Input: part model. Units: mm. Frame: model coordinates. Face numbers are marked on the shaded views. Coordinates: 2 decimals unless noted, no trailing zeros. Loops run counter-clockwise (first coordinate to the right, second up) from the corner with the lowest first, then second, coordinate; pieces in that order, holes last.
(1) Section C-C, the plane y = 4. Return loops of the section in (x, z).
(2) Line query: L1, parallel to X at y = 6.5, z = 0; L2, parallel to Z at x = 41, y = 5.25; L3, parallel to Z at x = 16.5, y = 4.75. Output: solid intervals per line, ascending.
(3) Contact query for flat-ended pins moving along their axis: P1, Ø1.5, axis at x = 13.5, y = 2.5, coming from the +Z side; P2, Ø2, axis at x = 41, z = 0, coming from the +Y side; P3, Ø5, axis at y = 7, z = 2, coming from the -X side; P4, Ø3, axis at x = -14.5, y = 3, coming from the -Z side. Output: stop coordinate, or through.
(4) Section B-B, the plane x = -14.5. Return loops of the section in (y, z), then the cut area to 3 significant figures.
(5) Mould query, pull axis X, two halves, no side actions, for the marked faces 1, 2 and 3. Classes: released by +X, released by -X, zero draft, split by the parting line, or undercut.
(6) Section A-A, the plane z = -16. Return loops of the section in (x, y).
(7) Section D-D, the plane x = -41. Return loops of the section in (y, z).
```python
from build123d import *

# Parameters (mm, degrees)
SCHIZZO1_R                             = 47
SCHIZZO1_R_2                           = 35
ESTRUSIONE_ESTRUSIONE1_DEPTH           = 10
FORO_SVASATO_PER_VITE_M3_1_D           = 3.4
FORO_SVASATO_PER_VITE_M3_1_DEPTH       = 188
FORO_SVASATO_PER_VITE_M3_1_CSINK_D     = 6.3
FORO_SVASATO_PER_VITE_M3_1_CSINK_ANGLE = 90
FORO_SVASATO_PER_VITE_M3_1_TIP         = 1.021463052


with BuildPart() as part:
    # Schizzo1 → Estrusione-Estrusione1 (new body)
    with BuildSketch(Plane(origin=(0, 0, 0), x_dir=(1, 0, 0), z_dir=(0, 1, 0))):
        with Locations(Location((0, 0, 0), (0, 0, 270))):
            Circle(SCHIZZO1_R)
        with Locations(Location((0, 0, 0), (0, 0, 270))):
            Circle(SCHIZZO1_R_2, mode=Mode.SUBTRACT)
    extrude(amount=ESTRUSIONE_ESTRUSIONE1_DEPTH)

    # Foro svasato per Vite M3-1
    with Locations(Plane(origin=(-41, 10, 0), x_dir=(0, 0, 1), z_dir=(0, 1, 0))):
        with Locations((0, 0), (0, 82), (41, 41), (-41, 41)):
            CounterSinkHole(FORO_SVASATO_PER_VITE_M3_1_D / 2, FORO_SVASATO_PER_VITE_M3_1_CSINK_D / 2, depth=FORO_SVASATO_PER_VITE_M3_1_DEPTH, counter_sink_angle=FORO_SVASATO_PER_VITE_M3_1_CSINK_ANGLE)
            with Locations((0, 0, -(FORO_SVASATO_PER_VITE_M3_1_DEPTH + FORO_SVASATO_PER_VITE_M3_1_TIP / 2))):  # 118° drill point
                Cone(0, FORO_SVASATO_PER_VITE_M3_1_D / 2, FORO_SVASATO_PER_VITE_M3_1_TIP, mode=Mode.SUBTRACT)


solid = part.part
```
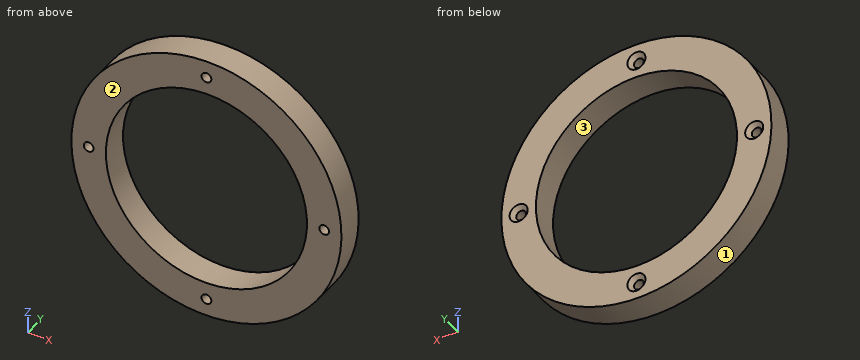
Report:
1. outline: circle Ø94 at (0, 0); hole circle Ø3.4 at (-41, 0); hole circle Ø70 at (0, 0); hole circle Ø3.4 at (0, -41); hole circle Ø3.4 at (0, 41); hole circle Ø3.4 at (41, 0)
2. L1: x = -47 to -42.7, -39.3 to -35, 35 to 39.3, 42.7 to 47
2. L2: z = -22.98 to -1.7, 1.7 to 22.98
2. L3: z = -44.01 to -30.87, 30.87 to 44.01
3. P1: stops at z = 45.24
3. P2: passes through
3. P3: stops at x = -47
3. P4: stops at z = -45.17
4. outline: (0, -44.71) - (10, -44.71) - (10, -31.86) - (0, -31.86) - close; (0, 31.86) - (10, 31.86) - (10, 44.71) - (0, 44.71) - close
4. area: 257 mm2
5. face 1: split by the parting line
5. face 2: zero draft
5. face 3: undercut
6. outline: (-44.19, 0) - (-31.13, 0) - (-31.13, 10) - (-44.19, 10) - close; (31.13, 0) - (44.19, 0) - (44.19, 10) - (31.13, 10) - close
7. outline: (0, -22.98) - (10, -22.98) - (10, -3.15) - (8.55, -1.7) - (0, -1.7) - close; (0, 1.7) - (8.55, 1.7) - (10, 3.15) - (10, 22.98) - (0, 22.98) - close
